```python
from build123d import *

# Parameters (mm, degrees)
F0_W           = 92.964
F0_H           = 111.76
F1_DEPTH       = 5.08
F3_D           = 4.4
F3_DEPTH       = 37.1856
F3_CSINK_D     = 8.96
F3_CSINK_ANGLE = 90
F3_TIP         = 1.3218933619


with BuildPart() as f1:
    # F0 (on Top) → F1 (new body)
    with BuildSketch(Plane.XY):
        Rectangle(F0_W, F0_H)
    extrude(amount=F1_DEPTH)

    # F3
    with Locations(Plane.XY.offset(5.08)):
        with Locations((-31.20898, 39.59098), (-31.20898, -39.58844), (31.27502, -39.58844), (31.27502, 39.59098)):
            CounterSinkHole(F3_D / 2, F3_CSINK_D / 2, depth=F3_DEPTH, counter_sink_angle=F3_CSINK_ANGLE)
            with Locations((0, 0, -(F3_DEPTH + F3_TIP / 2))):  # 118° drill point
                Cone(0, F3_D / 2, F3_TIP, mode=Mode.SUBTRACT)


solid = f1.part
```
The listing builds one solid part. Answer for the finished solid, in the listing's coordinates (mm). Give positions to 0.01 mm unless a question says otherwise; leave off trailing zeros. Write each loop counter-clockwise with the first axis right and the second up, starting at its lowest first coordinate (ties: lowest second). Pieces come first, ordered by that corner, then holes. Notation, with made-up numbers: (-8, 76.5) -> (35, 76.5) arc R8 cw to (35, 89.5) -> close; hole circle Ø1 at (46, 15.5). An arc over 180 degrees is marked (long way). Write item = value, one per line. Start each with the question number.
1) The part is cut by section A-A, the plane z = 4.25. Determine the outline of the cut face in (x, y), and give its area (3 significant figures).
2) Straight lines are drawn through the part: line 1 along Y through (x, z) = (-31, 2.35); line 2 along X through (y, z) = (-42, 4.5); line 3 along X through (y, z) = (-38, 2.9). For each, find the intervals that lie inside material, in ascending order.
3) Determine the mould class of faces 1 (the face through (-46.482, -1, 3)), 2 (the face through (-1, -55.88, 3)), 3 (the face through (-1, 55.88, 3)), 4 (the face through (33.109, 38.185, 2.911)) for opening direction Y: +Y half, -Y half, draft (parallel to the pull), parting line (faces both ways), or undercut.
4) Each of these flat-tipped pins is pushed along its axis until it touches: pin 1 (5.5 mm diameter, centred on x = -31.21, y = -39.59, fed in from +Z); pin 2 (2.5 mm diameter, centred on x = 31.28, y = -39.59, fed in from +Z). Where does it stop, or does it pass through?
Solutions:
q1.outline = (-46.48, -55.88) -> (46.48, -55.88) -> (46.48, 55.88) -> (-46.48, 55.88) -> close; hole circle Ø7.3 at (-31.21, -39.59); hole circle Ø7.3 at (-31.21, 39.59); hole circle Ø7.3 at (31.28, -39.59); hole circle Ø7.3 at (31.28, 39.59)
q1.area = 10,200 mm²
q2.line_1 = -55.88 to -41.78, -37.4 to 37.4, 41.78 to 55.88
q2.line_2 = -46.48 to -34.27, -28.14 to 28.21, 34.34 to 46.48
q2.line_3 = -46.48 to -32.87, -29.55 to 29.61, 32.94 to 46.48
q3.face_1 = draft
q3.face_2 = -Y half
q3.face_3 = +Y half
q3.face_4 = undercut
q4.pin_1 = 3.35
q4.pin_2 = through
